from build123d import *

# Parameters (mm, degrees)
SKETCH1_W           = 85
SKETCH1_H           = 85
SKETCH1_R           = 11.25
SKETCH1_R_2         = 2.25
BOSS_EXTRUDE1_DEPTH = 4


with BuildPart() as part:
    # Sketch1 → Boss-Extrude1 (new body)
    with BuildSketch(Plane(origin=(0, 0, 0), x_dir=(1, 0, 0), z_dir=(0, 1, 0))):
        with Locations((-7.5, 7.5)):
            Rectangle(SKETCH1_W, SKETCH1_H)
        Circle(SKETCH1_R, mode=Mode.SUBTRACT)
        with Locations((-15, 40)):
            Circle(SKETCH1_R_2, mode=Mode.SUBTRACT)
        with Locations((-40, 15)):
            Circle(SKETCH1_R_2, mode=Mode.SUBTRACT)
    extrude(amount=BOSS_EXTRUDE1_DEPTH)


solid = part.part
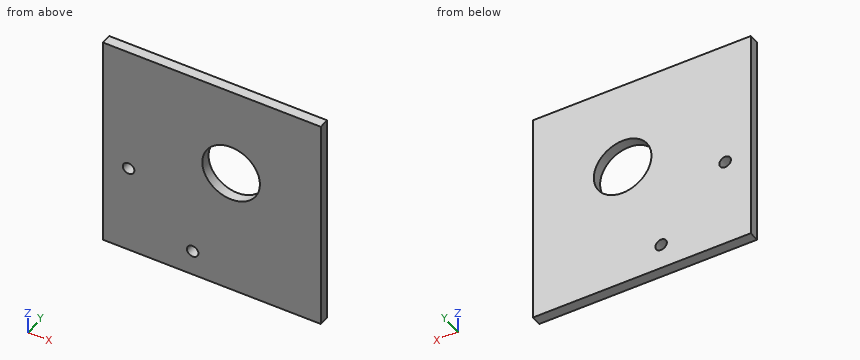
Input: part model. Units: mm. Frame: model coordinates. Coordinates: 2 decimals unless noted, no trailing zeros. Loops run counter-clockwise (first coordinate to the right, second up) from the corner with the lowest first, then second, coordinate; pieces in that order, holes last. Notation, with made-up numbers: (65, 58.5) -> (95, 58.5) arc R15 ccw to (95, 77.5) -> close; hole circle Ø6 at (56, 72.25). An arc over 180 degrees is marked (long way). One line per item, written item: value.
(1) Cut plane A-A (x = -40). Output: boundary loops of the cut face in (y, z), then the cut area to 3 significant figures.
Answer below:
outline: (0, -50) -> (4, -50) -> (4, -17.25) -> (0, -17.25) -> close; (0, -12.75) -> (4, -12.75) -> (4, 35) -> (0, 35) -> close
area: 322 mm2
(2) Ray query, line 1 along Z through (x, y) = (0, 1.05); line 2 along Z through (x, y) = (-40, 2.7); line 3 along X through (y, z) = (1.6, -15). Return the intervals inside material, ascending.
Answer below:
line 1: z = -50 to -11.25, 11.25 to 35
line 2: z = -50 to -17.25, -12.75 to 35
line 3: x = -50 to -42.25, -37.75 to 35
(3) Cut plane B-B (z = 0). Output: boundary loops of the cut face in (x, y), then the cut area to 3 significant figures.
Answer below:
outline: (-50, 0) -> (-11.25, 0) -> (-11.25, 4) -> (-50, 4) -> close; (11.25, 0) -> (35, 0) -> (35, 4) -> (11.25, 4) -> close
area: 250 mm2
(4) Cut plane C-C (y = 3.1). Output: boundary loops of the cut face in (x, z).
Answer below:
outline: (-50, -50) -> (35, -50) -> (35, 35) -> (-50, 35) -> close; hole circle Ø4.5 at (-40, -15); hole circle Ø4.5 at (-15, -40); hole circle Ø22.5 at (0, 0)
